Read the model definition and answer for the solid it produces. Units are mm, in the model's axes. Face numbers are marked on the shaded views. A direction names the side the tool comes from. Give positions to 0.01 mm unless a question says otherwise; leave off trailing zeros. Write each loop counter-clockwise with the first axis right and the second up, starting at its lowest first coordinate (ties: lowest second). Pieces come first, ordered by that corner, then holes. Notation, with made-up numbers: M -2.5,3.25 L 41.5,3.25 A31 cw 41.5,29.25 Z; hole C 85,85 d2. An arc over 180 degrees is marked long. Use a Markdown table: item, result. Add a question column.
Item 1: For the marked faces 1 and 2, determine the directions among +Z, -Z, +X, -X, +Y, -Y from which every point of the face is accessible in a straight line to the end or side of a thin tool.
Item 2: A cutting plane is placed at C-C on x = -109. Determine the outline of the cut face in (y, z).
Item 3: Given P1, Ø2, axis at x = 54, y = -203, coming from the +Z side; P2, Ø4, axis at y = -31, z = 185.5, coming from the -X side; P3, Ø10, axis at x = -257.5, y = -315.5, coming from the +Z side, each flat-ended and moving along its own axis, determine where each tip first touches the part or whether it passes through.
Item 4: Consider probe 1 along X at (y, z) = (410.5, -12); probe 2 along Z at (x, y) = (19.5, -355.5); probe 3 along Z at (x, y) = (-238, -237.5). Determine where each line is inside the solid, lowest interval first. Write a range as [from, to].
Item 5: A cutting plane is placed at B-B on z = 168.5. Determine the outline of the cut face in (x, y), then the cut area to 3 significant figures.
Item 6: A cutting plane is placed at A-A on y = -148. Determine the outline of the cut face in (x, z), then the cut area to 3 significant figures.
from build123d import *

# Parameters (mm, degrees)
F0_W          = 450
F0_H          = 50
F1_DEPTH      = 500
F1_DEPTH_BACK = 500


with BuildPart() as f1:
    # F0 (on Front) → F1 (new body, two sides)
    with BuildSketch(Plane.XZ) as f1_sk:
        Polygon((-20.51137, 356.582467), (-20.51137, -43.417533), (429.48863, -43.417533), (429.48863, 556.582467), (83.904198, 556.582467), (-450.51137, 426.582467), (-450.51137, 356.582467), align=None)
        with Locations((204.48863, -68.417533)):
            Rectangle(F0_W, F0_H)
    extrude(amount=F1_DEPTH)
    extrude(f1_sk.sketch, amount=-F1_DEPTH_BACK)


solid = f1.part
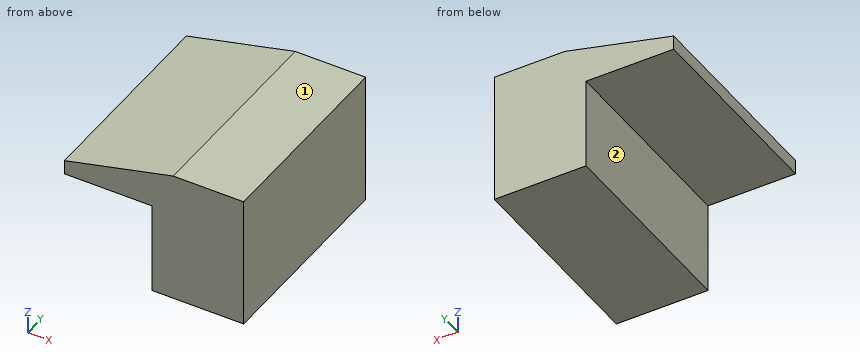
Filled in:
| question | item | result |
|---|---|---|
| 1 | face 1 | +Z, +X, -X, +Y, -Y |
| 1 | face 2 | -Z, -X, +Y, -Y |
| 2 | outline | M -500,356.58 L 500,356.58 L 500,509.66 L -500,509.66 Z |
| 3 | P1 | z = 549.55 |
| 3 | P2 | x = -20.51 |
| 3 | P3 | z = 474.75 |
| 4 | probe 1 | [-20.51, 429.49] |
| 4 | probe 2 | [-93.42, 540.92] |
| 4 | probe 3 | [356.58, 478.28] |
| 5 | outline | M -20.51,-500 L 429.49,-500 L 429.49,500 L -20.51,500 Z |
| 5 | area | 450,000 mm² |
| 6 | outline | M -450.51,356.58 L -20.51,356.58 L -20.51,-93.42 L 429.49,-93.42 L 429.49,556.58 L 83.9,556.58 L -450.51,426.58 Z |
| 6 | area | 344,000 mm² |
